Input: part model. Units: mm. Frame: model coordinates. A direction names the side the tool comes from. Coordinates: 2 decimals unless noted, no trailing zeros. Order: outer loops, then holes, each group sorted by start corner. A loop starts at its lowest first (then second) coordinate and runs counter-clockwise, first axis right, second up.
from build123d import *

# Parameters (mm, degrees)
F1_DEPTH = 15


with BuildPart() as f1:
    # F0 (on Top) → F1 (new body)
    with BuildSketch(Plane.XY):
        with BuildLine():
            ThreePointArc((20.5, -17.5), (19.62132, -19.62132), (17.5, -20.5))
            Line((17.5, -20.5), (-17.5, -20.5))
            ThreePointArc((-17.5, -20.5), (-19.62132, -19.62132), (-20.5, -17.5))
            Line((-20.5, -17.5), (-25.5, -17.5))
            ThreePointArc((-25.5, -17.5), (-34.5, -26.5), (-43.5, -17.5))
            Line((-43.5, -17.5), (-48.5, -17.5))
            ThreePointArc((-48.5, -17.5), (-39.503095, -30.575513), (-24.075852, -26.845433))
            ThreePointArc((-24.075852, -26.845433), (-21.875021, -25.420392), (-19.255656, -25.304977))
            ThreePointArc((-19.255656, -25.304977), (-18.383227, -25.451095), (-17.5, -25.5))
            Line((-17.5, -25.5), (17.5, -25.5))
            ThreePointArc((17.5, -25.5), (23.156854, -23.156854), (25.5, -17.5))
            Line((25.5, -17.5), (25.5, 17.5))
            ThreePointArc((25.5, 17.5), (23.156854, 23.156854), (17.5, 25.5))
            Line((17.5, 25.5), (-17.5, 25.5))
            ThreePointArc((-17.5, 25.5), (-23.156854, 23.156854), (-25.5, 17.5))
            Line((-25.5, 17.5), (-25.5, 9.074176))
            ThreePointArc((-25.5, 9.074176), (-27.358596, 5.184242), (-31.552632, 4.186235))
            ThreePointArc((-31.552632, 4.186235), (-43.295932, 1.391812), (-48.5, -9.5))
            Line((-48.5, -9.5), (-43.5, -9.5))
            ThreePointArc((-43.5, -9.5), (-34.5, -0.5), (-25.5, -9.5))
            Line((-25.5, -9.5), (-20.5, -9.5))
            Line((-20.5, -9.5), (-20.5, 17.5))
            ThreePointArc((-20.5, 17.5), (-19.62132, 19.62132), (-17.5, 20.5))
            Line((-17.5, 20.5), (17.5, 20.5))
            ThreePointArc((17.5, 20.5), (19.62132, 19.62132), (20.5, 17.5))
            Line((20.5, 17.5), (20.5, -17.5))
        make_face()
    extrude(amount=F1_DEPTH)


solid = f1.part
Item 1: Pin query (flat end, axial travel): pin 1 Ø7.5 at (x, z) = (-4, 8) entering from -Y; pin 2 Ø5.5 at (x, z) = (-22, 7) entering from +Y; pin 3 Ø2.5 at (x, z) = (-46, 6.5) entering from +Y; pin 4 Ø1.5 at (x, y) = (-26.5, -16) entering from -Z. Return the tip coordinate at first contact, or that it passes through.
Response values:
pin 1: stops at y = -25.5
pin 2: stops at y = 25.31
pin 3: stops at y = 0.04
pin 4: passes through
Item 2: Cut plane C-C on z = 12. Return loops of the section in (x, y).
Response values:
outline: (-48.5, -17.5) arc R14 ccw to (-24.08, -26.85) arc R5 cw to (-19.26, -25.3) arc R8 ccw to (-17.5, -25.5) - (17.5, -25.5) arc R8 ccw to (25.5, -17.5) - (25.5, 17.5) arc R8 ccw to (17.5, 25.5) - (-17.5, 25.5) arc R8 ccw to (-25.5, 17.5) - (-25.5, 9.07) arc R5 cw to (-31.55, 4.19) arc R14 ccw to (-48.5, -9.5) - (-43.5, -9.5) arc R9 cw to (-25.5, -9.5) - (-20.5, -9.5) - (-20.5, 17.5) arc R3 cw to (-17.5, 20.5) - (17.5, 20.5) arc R3 cw to (20.5, 17.5) - (20.5, -17.5) arc R3 cw to (17.5, -20.5) - (-17.5, -20.5) arc R3 cw to (-20.5, -17.5) - (-25.5, -17.5) arc R9 cw to (-43.5, -17.5) - close
Item 3: Draft query along X for faces 6 (the face through (-23.094, 23.219, 7.395)), 7 (the face through (0, -20.5, 7)), 8 (the face through (-23, -5, 15)). Return one class per face: pulls with the +X half, pulls with the -X half, needs draft (parallel to the pull), parting line crosses it, or undercut.
Response values:
face 6: pulls with the -X half
face 7: undercut
face 8: needs draft
Item 4: Ray query, probe 1 along Y at (x, z) = (7, 2.75); probe 2 along X at (y, z) = (-18, 7); probe 3 along X at (y, z) = (-8, 12). Return the intervals inside material, ascending.
Response values:
probe 1: y = -25.5 to -20.5, 20.5 to 25.5
probe 2: x = -48.49 to -43.49, -25.51 to -20.46, 20.46 to 25.48
probe 3: x = -48.42 to -43.37, -25.63 to -20.5, 20.5 to 25.5
Item 5: Cut plane B-B on y = 1. Return loops of the section in (x, z).
Response values:
outline: (-43.76, 0) - (-20.5, 0) - (-20.5, 15) - (-43.76, 15) - close; (20.5, 0) - (25.5, 0) - (25.5, 15) - (20.5, 15) - close
Item 6: Access query for faces 1 (the face through (-25.5, 13, 7)), 2 (the face through (-46, -9.5, 7)), 3 (the face through (-34.698, -0.502, 7.395)), 4 (the face through (0, 25.5, 7)), 5 (the face through (0, -25.5, 7)). Directions: +Z, -Z, +X, -X, +Y, -Y. A direction counts if a zero-diameter tool reaches every point of the face in a straight line with its end or side. Return the directions, or none.
Response values:
face 1: +Z, -Z, -X, +Y
face 2: +Z, -Z, -X
face 3: +Z, -Z
face 4: +Z, -Z, +X, -X, +Y
face 5: +Z, -Z, +X, -Y
Item 7: Cut plane A-A on x = -34.5. Return loops of the section in (y, z), then the cut area to 3 significant figures.
Response values:
outline: (-31.5, 0) - (-26.5, 0) - (-26.5, 15) - (-31.5, 15) - close; (-0.5, 0) - (4.5, 0) - (4.5, 15) - (-0.5, 15) - close
area: 150 mm2
